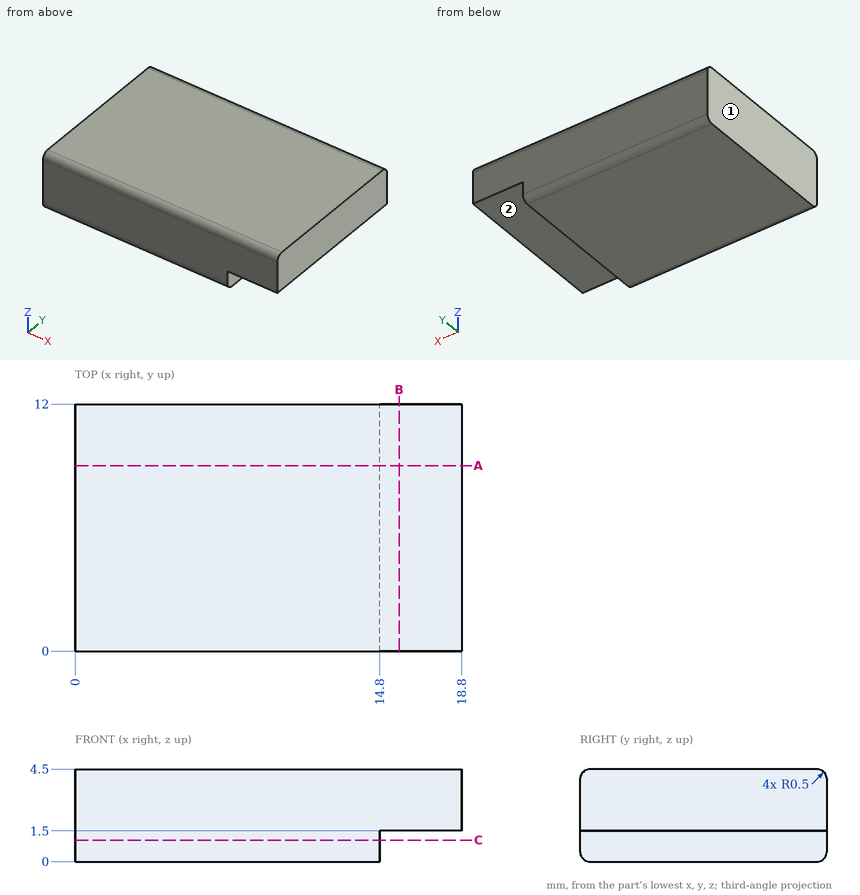
Part print with two shaded views. Sizes in mm from the minimum x, y, z corner. A direction names the side the tool comes from. Round coordinates to 2 decimals unless told otherwise and drop trailing zeros. Order: outer loops, then holes, each group sorted by start corner. A loop starts at its lowest first (then second) coordinate and runs counter-clockwise, first axis right, second up. Notation, with made-up numbers: M 36,69 L 57,69 A12 ccw 57,78 Z; hole C 67.5,2 d10. An arc over 180 degrees is marked long. Answer in a Markdown table with one row per item. Add a question column.
Q1. Cut at C-C on z = 1.05. Give the cut face in (x, y).
Q2. Wall check: L1, parallel to X at y = 8, z = 1.4. Give the ranges that are in metal, low to high. Write a range as from..to.
Q3. Pin check, flat tip, straight feed: pin 1 (0.8 mm diameter, centred on y = 4, z = 1, fed in from +X). Stop position of the tip, or through.
Q4. 3-axis set-ups, long thin cutter, end or side, ignore diameter. For the marked faces 1 and 2: which of +Z, -Z, +X, -X, +Y, -Y reach the whole face in a straight line?
Q5. Cut at A-A on y = 9. Give the cut face in (x, z), and give its area (3 significant figures).
Q6. Cut at B-B on x = 15.75. Give the cut face in (y, z).
Established:
| question | item | result |
|---|---|---|
| 1 | outline | M 0,0 L 14.8,0 L 14.8,12 L 0,12 Z |
| 2 | L1 | x = 0..14.8 |
| 3 | pin 1 | stops at x = 14.8 |
| 4 | face 1 | +Z, -Z, -X, +Y, -Y |
| 4 | face 2 | -Z, +X, +Y, -Y |
| 5 | outline | M 0,0 L 14.8,0 L 14.8,1.5 L 18.8,1.5 L 18.8,4.5 L 0,4.5 Z |
| 5 | area | 78.6 mm2 |
| 6 | outline | M 0,1.5 L 12,1.5 L 12,4 A0.5 ccw 11.5,4.5 L 0.5,4.5 A0.5 ccw 0,4 Z |
